Could you check a few things on this model? Use its own coordinates, in mm. Face numbers are marked on the shaded views. A direction names the side the tool comes from. Give positions to 0.01 mm unless a question says otherwise; leave off trailing zeros. Loops run counter-clockwise (first coordinate to the right, second up) from the corner with the lowest first, then second, coordinate; pieces in that order, holes last. Notation, with made-up numbers: (7, -27) - (39, -27) arc R33 ccw to (39, 1) - close; hole circle Ø6 at (44.5, 5.5). An arc over 180 degrees is marked (long way). Answer in a Markdown table with one row per item. Add a question column.
```python
from build123d import *

# Parameters (mm, degrees)
SKETCH_1_W          = 4
SKETCH_1_H          = 16
EXTRUDE_1_DEPTH     = 25
EXTRUDE_1_2_DEPTH   = 25
EXTRUDE_2_DEPTH     = 2.5
SKETCH_5_R          = 1.5
CUT_EXTRUDE_1_DEPTH = 42.496987842


with BuildPart() as part:
    # Sketch 1 → Extrude 1 (new body)
    with BuildSketch(Plane.XY):
        with Locations((-11, 0)):
            Rectangle(SKETCH_1_W, SKETCH_1_H)
    extrude(amount=EXTRUDE_1_DEPTH)



with BuildPart() as body_2:
    # Sketch 1 → Extrude 1 2 (new body)
    with BuildSketch(Plane.XY):
        Polygon((13, 6), (13, 8), (9, 8), (9, -8), (13, -8), (13, -6), align=None)
    extrude(amount=EXTRUDE_1_2_DEPTH)


with BuildPart() as part_1:
    add(part.part)

    add(body_2.part)  # Extrude 2 merges body 2
    # Sketch 1_4 → Extrude 2 (add)
    with BuildSketch(Plane.XY):
        with BuildLine():
            Line((-9.539392014, 13), (-11.5, 13))
            ThreePointArc((-11.5, 13), (-11.939339828, 11.939339828), (-13, 11.5))
            Line((-13, 11.5), (-13, 8))
            Line((-13, 8), (-9, 8))
            Line((-9, 8), (-9, -8))
            Line((-9, -8), (-13, -8))
            Line((-13, -8), (-13, -11.5))
            ThreePointArc((-13, -11.5), (-11.939339828, -11.939339828), (-11.5, -13))
            Line((-11.5, -13), (-9.539392014, -13))
            ThreePointArc((-9.539392014, -13), (0, -6), (9.539392014, -13))
            Line((9.539392014, -13), (11.5, -13))
            ThreePointArc((11.5, -13), (11.939339828, -11.939339828), (13, -11.5))
            Line((13, -11.5), (13, -8))
            Line((13, -8), (9, -8))
            Line((9, -8), (9, 8))
            Line((9, 8), (13, 8))
            Line((13, 8), (13, 11.5))
            ThreePointArc((13, 11.5), (11.939339828, 11.939339828), (11.5, 13))
            Line((11.5, 13), (9.539392014, 13))
            ThreePointArc((9.539392014, 13), (0, 6), (-9.539392014, 13))
        make_face()
        with BuildLine():
            ThreePointArc((-13, 11.5), (-14.060660172, 14.060660172), (-11.5, 13))
            Line((-11.5, 13), (-9.539392014, 13))
            ThreePointArc((-9.539392014, 13), (-9.884177258, 14.482423007), (-10, 16))
            Line((-10, 16), (-13, 16))
            ThreePointArc((-13, 16), (-15.121320344, 15.121320344), (-16, 13))
            Line((-16, 13), (-16, -13))
            ThreePointArc((-16, -13), (-15.121320344, -15.121320344), (-13, -16))
            Line((-13, -16), (-10, -16))
            ThreePointArc((-10, -16), (-9.884177258, -14.482423007), (-9.539392014, -13))
            Line((-9.539392014, -13), (-11.5, -13))
            ThreePointArc((-11.5, -13), (-14.060660172, -14.060660172), (-13, -11.5))
            Line((-13, -11.5), (-13, -8))
            Line((-13, -8), (-13, 8))
            Line((-13, 8), (-13, 11.5))
        make_face()
        with BuildLine():
            ThreePointArc((10, 16), (9.884177258, 14.482423007), (9.539392014, 13))
            Line((9.539392014, 13), (11.5, 13))
            ThreePointArc((11.5, 13), (13, 14.5), (14.5, 13))
            ThreePointArc((14.5, 13), (14.060660172, 11.939339828), (13, 11.5))
            Line((13, 11.5), (13, 8))
            Line((13, 8), (13, 6))
            Line((13, 6), (13, -6))
            Line((13, -6), (13, -8))
            Line((13, -8), (13, -11.5))
            ThreePointArc((13, -11.5), (14.060660172, -11.939339828), (14.5, -13))
            ThreePointArc((14.5, -13), (13, -14.5), (11.5, -13))
            Line((11.5, -13), (9.539392014, -13))
            ThreePointArc((9.539392014, -13), (9.884177258, -14.482423007), (10, -16))
            Line((10, -16), (13, -16))
            ThreePointArc((13, -16), (15.121320344, -15.121320344), (16, -13))
            Line((16, -13), (16, 13))
            ThreePointArc((16, 13), (15.121320344, 15.121320344), (13, 16))
            Line((13, 16), (10, 16))
        make_face()
    extrude(amount=EXTRUDE_2_DEPTH)

    # Sketch 5 → Cut-Extrude 1 (cut, through all)
    with BuildSketch(Plane.ZY.offset(13)):
        Polygon((25, 8), (2.5, 8), (22.464054272, 2.90689625), (25, 2.259941753), align=None)
        Polygon((25, -2.259941753), (22.464054353, -2.906896229), (2.5, -8), (25, -8), align=None)
        with BuildLine():
            Line((25, 2.259941753), (22.464054272, 2.90689625))
            ThreePointArc((22.464054272, 2.90689625), (24.091512257, 1.840547895), (24.722465308, 0))
            ThreePointArc((24.722465308, 0), (24.091512283, -1.840547862), (22.464054353, -2.906896229))
            Line((22.464054353, -2.906896229), (25, -2.259941753))
            Line((25, -2.259941753), (25, 2.259941753))
        make_face()
        with Locations(Location((21.722465308, 0, 0), (0, 0, 90))):
            Circle(SKETCH_5_R)
    extrude(amount=-CUT_EXTRUDE_1_DEPTH, mode=Mode.SUBTRACT)


solid = part_1.part
```
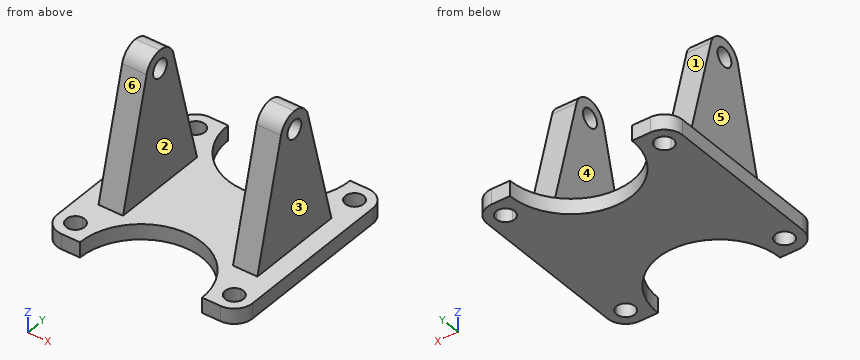
(1) Please list where these lines run through material, in increasing order: line 1 (Y direction, x = 13, z = 2.25); line 2 (X direction, y = -13, z = 1.2); line 3 (X direction, y = 1, z = 9.75).
(2) For pin 1 Ø13 at (y, z) = (-1.5, 15.5) entering from -X; pin 2 Ø13 at (y, z) = (-1, 15.5) entering from +X; pin 3 Ø6 at (x, z) = (9.5, 12) entering from +Y, each with a flat end and sliding along its axis, tell me the tip position at first contact or that it passes through.
(3) I want a section at B-B on z = 14.25. Please give me the cut outline in (x, y).
(4) I want a section at A-A on x = 12. Please give me the cut outline in (y, z).
(5) I want a section at C-C on y = 11. Please give me the cut outline in (x, z).
(6) We'd pull the mould along X, two halves only. Please class the marked faces 4, 5 and 6: pulls with the +X half, pulls with the -X half, needs draft (parallel to the pull), parting line crosses it, or undercut.
(7) I want a section at D-D on z = 21. Please give me the cut outline in (x, y).
(8) On a 3-axis mill with a long thin cutter (end or side, diameter ignored), from which of +Z, -Z, +X, -X, +Y, -Y can I reach the whole of each face in a straight line? I mean the marked faces 1, 2 and 3. Say none if no direction works.
Reported:
| question | item | result |
|---|---|---|
| 1 | line 1 | -16 to -14.5, -11.5 to 11.5, 14.5 to 16 |
| 1 | line 2 | -16 to -14.5, -11.5 to -9.54, 9.54 to 11.5, 14.5 to 16 |
| 1 | line 3 | -13 to -9, 9 to 13 |
| 2 | pin 1 | x = -13 |
| 2 | pin 2 | x = 13 |
| 2 | pin 3 | y = 6.34 |
| 3 | outline | (-13, -5) - (-9, -5) - (-9, 5) - (-13, 5) - close; (9, -5) - (13, -5) - (13, 5) - (9, 5) - close |
| 4 | outline | (-16, 0) - (-14.12, 0) - (-14.12, 2.5) - (-16, 2.5) - close; (-11.88, 0) - (11.88, 0) - (11.88, 2.5) - (8, 2.5) - (2.91, 22.46) arc R3 ccw to (-2.91, 22.46) - (-8, 2.5) - (-11.88, 2.5) - close; (14.12, 0) - (16, 0) - (16, 2.5) - (14.12, 2.5) - close; hole circle Ø3 at (0, 21.72) |
| 5 | outline | (-16, 0) - (-8.66, 0) - (-8.66, 2.5) - (-16, 2.5) - close; (8.66, 0) - (16, 0) - (16, 2.5) - (8.66, 2.5) - close |
| 6 | face 4 | undercut |
| 6 | face 5 | pulls with the -X half |
| 6 | face 6 | needs draft |
| 7 | outline | (-13, -3.28) - (-9, -3.28) - (-9, -1.31) - (-13, -1.31) - close; (-13, 1.31) - (-9, 1.31) - (-9, 3.28) - (-13, 3.28) - close; (9, -3.28) - (13, -3.28) - (13, -1.31) - (9, -1.31) - close; (9, 1.31) - (13, 1.31) - (13, 3.28) - (9, 3.28) - close |
| 8 | face 1 | +Z, +X, -X, +Y |
| 8 | face 2 | +Z, +Y, -Y |
| 8 | face 3 | +Z, +X, +Y, -Y |
